For this review, take the finished solid that the model builds, in its own axes (mm). Face numbers are marked on the shaded views. A direction names the side the tool comes from. Give positions to 0.01 mm unless a question says otherwise; leave off trailing zeros. Order: outer loops, then holes, each group sorted by start corner. A loop starts at its lowest first (then second) coordinate and runs counter-clockwise, first axis right, second up.
from build123d import *

# Parameters (mm, degrees)
EXTRUDE_1_DEPTH     = 7
SKETCH_3_R          = 3.56
CUT_EXTRUDE_1_DEPTH = 20
SKETCH_4_R          = 1.35
CUT_EXTRUDE_2_DEPTH = 14
FILLET_1_R          = 5
CHAMFER_1_SIZE      = 4


with BuildPart() as part:
    # 草图1 → 凸台-拉伸1 (new, symmetric)
    with BuildSketch(Plane.XY):
        Polygon((-7.5, -18), (7.5, -18), (7.5, 23), (7.5, 52), (-2.5, 52), (-2.5, 70), (-7.5, 70), (-7.5, 52), (-7.5, 47), align=None)
    extrude(amount=EXTRUDE_1_DEPTH, both=True)

    # 草图3 → 切除-拉伸1 (cut)
    with BuildSketch(Plane(origin=(7.5, 0, 0), x_dir=(0, 0, -1), z_dir=(1, 0, 0))):
        with Locations((0, -10)):
            Circle(SKETCH_3_R)
        with Locations((0, 10)):
            Circle(SKETCH_3_R)
    extrude(amount=-CUT_EXTRUDE_1_DEPTH, mode=Mode.SUBTRACT)

    # 草图4 → 切除-拉伸2 (cut)
    with BuildSketch(Plane.XY.offset(7)):
        Circle(SKETCH_4_R)
    extrude(amount=-CUT_EXTRUDE_2_DEPTH, mode=Mode.SUBTRACT)

    # 圆角1
    fillet_1_edges = [part.edges().sort_by_distance(p)[0] for p in [
        (-5, 70, 7),
        (-5, 70, -7),
    ]]
    fillet(fillet_1_edges, radius=FILLET_1_R)

    # 倒角1
    chamfer_1_edges = [part.edges().sort_by_distance(p)[0] for p in [
        (7.5, 52, 0),
    ]]
    chamfer(chamfer_1_edges, length=CHAMFER_1_SIZE)


solid = part.part
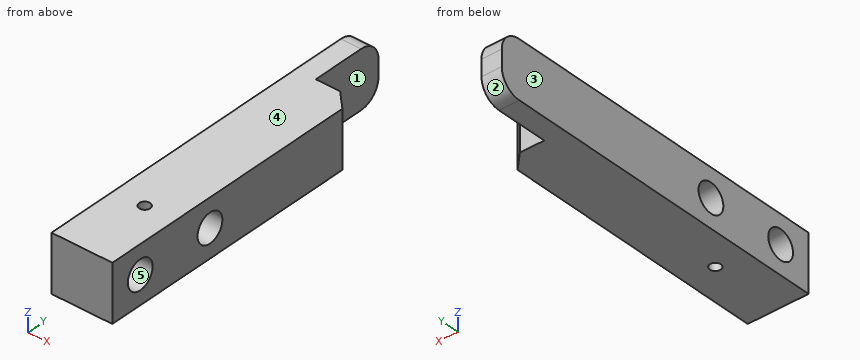
1) Clearance check with flat-ended pins moving along their axes: pin 1 (8 mm diameter, centred on x = 4, z = 5, fed in from +Y); pin 2 (1.6 mm diameter, centred on x = 0, y = 0, fed in from -Z); pin 3 (4 mm diameter, centred on y = 61.5, z = 1, fed in from +X); pin 4 (8 mm diameter, centred on y = 10, z = 0, fed in from +X). State where each tip first meets the part, or that it passes through.
Answer sheet:
pin 1: stops at y = 52
pin 2: passes through
pin 3: stops at x = -2.5
pin 4: stops at x = 7.5
2) Tool access review of the marked faces 1 and 2: name each direction out of +Z, -Z, +X, -X, +Y, -Y from which nothing blocks a thin tool from reaching the whole face with its end or side.
Answer sheet:
face 1: +Z, -Z, +X, +Y
face 2: -Z, +X, -X, +Y
3) We need section B-B on z = 0. Give the boundary of the cut face in (x, y).
Answer sheet:
outline: (-7.5, -18) - (7.5, -18) - (7.5, -13.56) - (-7.5, -13.56) - close; (-7.5, -6.44) - (7.5, -6.44) - (7.5, 6.44) - (-7.5, 6.44) - close; (-7.5, 13.56) - (7.5, 13.56) - (7.5, 48) - (3.5, 52) - (-2.5, 52) - (-2.5, 70) - (-7.5, 70) - close; hole circle Ø2.7 at (0, 0)
4) We need section C-C on y = 0. Give the boundary of the cut face in (x, z), then the cut area to 3 significant figures.
Answer sheet:
outline: (-7.5, -7) - (-1.35, -7) - (-1.35, 7) - (-7.5, 7) - close; (1.35, -7) - (7.5, -7) - (7.5, 7) - (1.35, 7) - close
area: 172 mm2
5) We need section A-A on x = 0. Give the boundary of the cut face in (y, z).
Answer sheet:
outline: (-18, -7) - (-1.35, -7) - (-1.35, 7) - (-18, 7) - close; (1.35, -7) - (52, -7) - (52, 7) - (1.35, 7) - close; hole circle Ø7.12 at (-10, 0); hole circle Ø7.12 at (10, 0)
6) To check wall thickness, follow line 1 (Y direction, x = 0.75, z = 1.5); line 2 (Y direction, x = 7.25, z = -3); line 3 (Y direction, x = 0.25, z = 0). State the ranges of each line that lie inside material, in increasing order.
Answer sheet:
line 1: y = -18 to -13.23, -6.77 to -1.12, 1.12 to 6.77, 13.23 to 52
line 2: y = -18 to -11.92, -8.08 to 8.08, 11.92 to 48.25
line 3: y = -18 to -13.56, -6.44 to -1.33, 1.33 to 6.44, 13.56 to 52
7) Draft analysis for pull direction Z (two halves, no side actions). For the marked faces 3, 4 and 5, state which applies: +Z half, -Z half, draft (parallel to the pull), parting line (faces both ways), or undercut.
Answer sheet:
face 3: draft
face 4: +Z half
face 5: undercut
8) We need section D-D on z = 6. Give the boundary of the cut face in (x, y), then the cut area to 3 significant figures.
Answer sheet:
outline: (-7.5, -18) - (7.5, -18) - (7.5, 48) - (3.5, 52) - (-2.5, 52) - (-2.5, 68) - (-7.5, 68) - close; hole circle Ø2.7 at (0, 0)
area: 1,120 mm2
